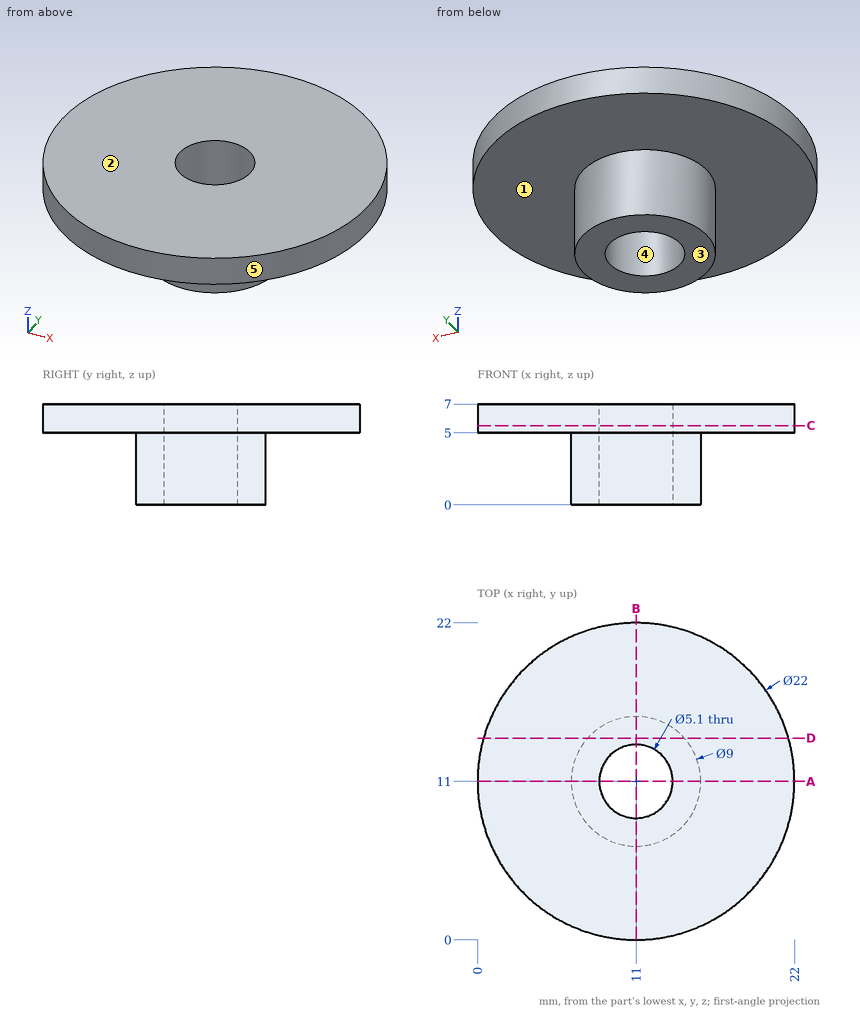
Design review of the part shown in the three views and the two pictorial views. Dimensions are in mm from the part's minimum x, y and z. A direction names the side the tool comes from. Give positions to 0.01 mm unless a question says otherwise; leave off trailing zeros. Loops run counter-clockwise (first coordinate to the right, second up) from the corner with the lowest first, then second, coordinate; pieces in that order, holes last. Notation, with made-up numbers: M 9.25,-35.5 L 65.25,-35.5 A20 cw 65.25,-10.5 Z; hole C 7,80 d11. An arc over 180 degrees is marked long. Put each result on its own line as item: value. Start each with the question number.
(1) For pin 1 (6.5 mm diameter, centred on x = 8.5, y = 12, fed in from -Z); pin 2 (3 mm diameter, centred on y = 14.5, z = 2.5, fed in from -X); pin 3 (4.5 mm diameter, centred on x = 11, y = 11, fed in from +Z), all flat-tipped, find the tip position at first contact; note any pin that passes through.
(2) Add section A-A, the plane y = 11. Write out the cut boundary in (x, z).
(3) Wall thickness on L1, parallel to Y at x = 11, z = 4.75; L2, parallel to Z at x = 14.75, y = 2.75; L3, parallel to X at y = 8.75, z = 3.25: over which ranges is each line inside the solid? List them lowest first.
(4) Add section D-D, the plane y = 14. Write out the cut boundary in (x, z), then the cut area to 3 significant figures.
(5) Add section C-C, the plane z = 5.5. Write out the cut boundary in (x, y).
(6) Machinability: for the marked faces 1 and 2, which of the approach directions +Z, -Z, +X, -X, +Y, -Y give a long, thin tool a straight path to every point of the face, cutting with its end or side? Answer none if there is none.
(7) The part is to be moulded in two halves that separate along X. For the marked faces 3, 4 and 5, say which applies: +X half, -X half, draft (parallel to the pull), parting line (faces both ways), or undercut.
Result:
1. pin 1: stops at z = 0
1. pin 2: stops at x = 6.97
1. pin 3: passes through
2. outline: M 0,5 L 6.5,5 L 6.5,0 L 8.45,0 L 8.45,7 L 0,7 Z; M 13.55,0 L 15.5,0 L 15.5,5 L 22,5 L 22,7 L 13.55,7 Z
3. L1: y = 6.5 to 8.45, 13.55 to 15.5
3. L2: z = 5 to 7
3. L3: x = 7.1 to 9.8, 12.2 to 14.9
4. outline: M 0.42,5 L 7.65,5 L 7.65,0 L 14.35,0 L 14.35,5 L 21.58,5 L 21.58,7 L 0.42,7 Z
4. area: 75.9 mm^2
5. outline: C 11,11 d22; hole C 11,11 d5.1
6. face 1: -Z
6. face 2: +Z, +X, -X, +Y, -Y
7. face 3: draft
7. face 4: undercut
7. face 5: parting line
